Geometry: final body of the model. Coordinates: model frame, mm. A direction names the side the tool comes from. Give positions to 0.01 mm unless a question says otherwise; leave off trailing zeros. Order: outer loops, then holes, each group sorted by start corner. A loop starts at its lowest first (then second) coordinate and runs counter-clockwise, first axis right, second up. Notation, with made-up numbers: (-20.5, 1.25) - (5.5, 1.25) arc R12 cw to (5.5, 17.25) - close; hole circle Ø3 at (9, 72). An arc over 180 degrees is marked (long way). Use one line per item in the form item = value.
from build123d import *

# Parameters (mm, degrees)
KES_EKSTR_ZYON1_START = -30
IZIM2_R               = 15.5
IZIM2_R_2             = 12.7
IZIM2_R_3             = 11.2
KES_EKSTR_ZYON1_DEPTH = 30
IZIM3_R               = 13.5
KES_EKSTR_ZYON2_DEPTH = 30


with BuildPart() as part:
    # Çizim1 → Döndür1 (revolve)
    with BuildSketch(Plane.XY, mode=Mode.PRIVATE) as d_nd_r1_sk:
        Polygon((-20.912241055, -5.436911488), (-20.912241055, 55.563088512), (-33.612241055, 55.563088512), (-33.612241055, 44.563088512), (-37.912241055, 44.563088512), (-37.912241055, 28.563088512), (-37.412241055, 28.563088512), (-37.412241055, 23.563088512), (-37.912241055, 23.563088512), (-37.912241055, 20.563088512), (-35.912241055, 20.563088512), (-35.912241055, -5.436911488), align=None)
    revolve(d_nd_r1_sk.sketch.rotate(Axis((-20.912241055, -5.436911488, 0), (0, 1, 0)), 270), axis=Axis((-20.912241055, -5.436911488, 0), (0, 1, 0)))

    # Çizim2 → Kes-Ekstrüzyon1 (cut)
    # profile 1 of 2: a face of its own
    with BuildSketch(Plane(origin=(0, 55.563088512, 0), x_dir=(1, 0, 0), z_dir=(0, 1, 0)).offset(KES_EKSTR_ZYON1_START)):
        with Locations(Location((-20.912241055, 0, 0), (0, 0, 270))):
            Circle(IZIM2_R)
        with Locations(Location((-20.912241055, 0, 0), (0, 0, 90))):
            Circle(IZIM2_R_2, mode=Mode.SUBTRACT)
    # profile 2 of 2: a face of its own
    with BuildSketch(Plane(origin=(0, 55.563088512, 0), x_dir=(1, 0, 0), z_dir=(0, 1, 0)).offset(KES_EKSTR_ZYON1_START)):
        with Locations(Location((-20.912241055, 0, 0), (0, 0, 270))):
            Circle(IZIM2_R_3)
    extrude(amount=KES_EKSTR_ZYON1_DEPTH, mode=Mode.SUBTRACT)

    # Çizim3 → Kes-Ekstrüzyon2 (cut)
    with BuildSketch(Plane.XZ.offset(5.436911488)):
        with Locations(Location((-20.912241055, 0, 0), (0, 0, 270))):
            Circle(IZIM3_R)
    extrude(amount=-KES_EKSTR_ZYON2_DEPTH, mode=Mode.SUBTRACT)


solid = part.part
(1) Cut plane D-D on y = 0. Output: boundary loops of the cut face in (x, z), plus the area to 3 significant figures.
Computed values:
outline = circle Ø30 at (-20.91, 0); hole circle Ø27 at (-20.91, 0)
area = 134 mm²
(2) Reachability of faces 1 (the face through (-35, 28.563, 9)), 2 (the face through (-31.846, 40.353, -2.428)), 3 (the face through (-11.78, 7.38, 11.9)), 4 (the face through (-4.316, 36.451, 3.685)), 5 (the face through (-29, -5.437, 11)) from +Z, -Z, +X, -X, +Y, -Y: full face, straight path, thin tool, end or side. Return the list, or none.
Computed values:
face_1 = none
face_2 = +Y
face_3 = -Y
face_4 = +Y, -Y
face_5 = +Z, -Z, +X, -X, -Y
(3) Cut plane C-C on y = 41.5. Output: boundary loops of the cut face in (x, z).
Computed values:
outline = circle Ø34 at (-20.91, 0); circle Ø25.4 at (-20.91, 0); hole circle Ø31 at (-20.91, 0); hole circle Ø22.4 at (-20.91, 0)
(4) Pull-direction query (Z, two-part tool) for faces 6 (the face through (-11.6, 55.563, 6.5)), 7 (the face through (-4.316, 22.042, 3.685)), 8 (the face through (-36.044, 34.93, -3.36)); classes: released by +Z, released by -Z, zero draft, split by the parting line, or undercut.
Computed values:
face_6 = zero draft
face_7 = split by the parting line
face_8 = undercut
(5) Contact query for flat-ended pins moving along their axis: pin 1 Ø4 at (x, z) = (-17.5, -7.5) entering from +Y; pin 2 Ø4 at (x, y) = (-19, 9.5) entering from +Z; pin 3 Ø1 at (y, z) = (23, -2) entering from +X. Output: stop coordinate, or through.
Computed values:
pin_1 = 25.56
pin_2 = 15
pin_3 = -3.98
(6) Ray query, line 1 along X through (y, z) = (32.25, 0); line 2 along X through (y, z) = (42, 5); line 3 along Z through (x, y) = (-17, 35). Return the intervals inside material, ascending.
Computed values:
line_1 = -37.91 to -36.41, -33.61 to -32.11, -9.71 to -8.21, -5.41 to -3.91
line_2 = -37.16 to -35.58, -32.59 to -30.93, -10.89 to -9.24, -6.24 to -4.66
line_3 = -16.54 to -15, -12.08 to -10.49, 10.49 to 12.08, 15 to 16.54
